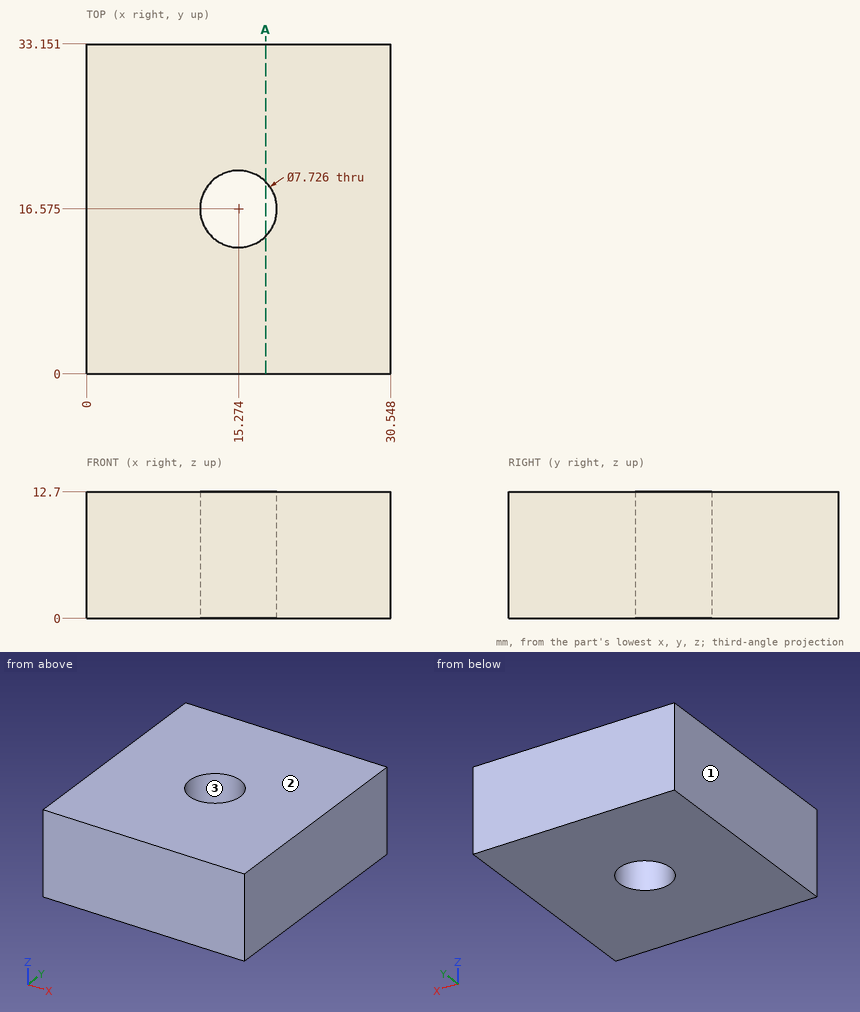
The figure shows three views and two pictorial views of one solid part (mm, origin at its lowest corner). Answer the questions. Give positions to 0.01 mm unless a question says otherwise; leave off trailing zeros. Loops run counter-clockwise (first coordinate to the right, second up) from the corner with the lowest first, then second, coordinate; pieces in that order, holes last. Notation, with made-up numbers: (-26.75, 23.25) -> (-16.75, 23.25) arc R31 ccw to (-16.75, 55.25) -> close; hole circle Ø7 at (77.25, 68). An arc over 180 degrees is marked (long way). Use CSV: the item, a comma, the result in double quotes.
1. The part is cut by section A-A (x = 18). Write down the section's boundary in (y, z).
Found:
outline,"(0, 0) -> (13.84, 0) -> (13.84, 12.7) -> (0, 12.7) -> close; (19.31, 0) -> (33.15, 0) -> (33.15, 12.7) -> (19.31, 12.7) -> close"
2. A flat-ended cylindrical pin translates along its axis: pin 1 Ø3 at (y, z) = (7, 10) entering from -X. Find the tip coordinate at first contact, or state that the pin passes through.
Found:
pin 1,"x = 0"
3. The mould has two halves that part along X. Classify the marked faces 1, 2 and 3: +X half, -X half, draft (parallel to the pull), parting line (faces both ways), or undercut.
Found:
face 1,"-X half"
face 2,"draft"
face 3,"undercut"
4. Straight lines are drawn through the part: line 1 (X direction, y = 15, z = 9.25); line 2 (Y direction, x = 17.5, z = 4.5); line 3 (X direction, y = 16, z = 4.75) (1 decimal). For each, find the intervals that lie inside material, in ascending order.
Found:
line 1,"0 to 11.75, 18.8 to 30.55"
line 2,"0 to 13.42, 19.73 to 33.15"
line 3,"0 to 11.5, 19.1 to 30.5"
